from build123d import *

# Parameters (mm, degrees)
SKETCH_W        = 6
SKETCH_H        = 29
SKETCH_R        = 1.65
PAD_DEPTH       = 2.7
SKETCH001_W     = 4.5
SKETCH001_H     = 29
PAD001_DEPTH    = 1.5
SKETCH002_R     = 1.65
POCKET_DEPTH    = 5.701
CHAMFER_SIZE    = 0.4
CHAMFER001_SIZE = 0.4
FILLET_R        = 1
FILLET001_R     = 1


with BuildPart() as part:
    # Sketch → Pad (new body)
    with BuildSketch(Plane.XY):
        with Locations((-0.5, -9.5)):
            Rectangle(SKETCH_W, SKETCH_H)
        Circle(SKETCH_R, mode=Mode.SUBTRACT)
        with Locations((0, -10)):
            Circle(SKETCH_R, mode=Mode.SUBTRACT)
        with Locations((0, -20)):
            Circle(SKETCH_R, mode=Mode.SUBTRACT)
    extrude(amount=PAD_DEPTH)

    # Sketch001 (on Face8 of Pad) → Pad001 (join)
    with BuildSketch(Plane(origin=(0, 0, 0), x_dir=(1, 0, 0), z_dir=(0, 0, -1))):
        with Locations((-1.25, 9.5)):
            Rectangle(SKETCH001_W, SKETCH001_H)
    extrude(amount=PAD001_DEPTH)

    # Sketch002 → Pocket (cut, through all)
    with BuildSketch(Plane.XY.offset(4.2)):
        Circle(SKETCH002_R)
        with Locations((0, -10)):
            Circle(SKETCH002_R)
        with Locations((0, -20)):
            Circle(SKETCH002_R)
    extrude(amount=-POCKET_DEPTH, mode=Mode.SUBTRACT)

    # Chamfer
    chamfer_edges = [part.edges().sort_by_distance(p)[0] for p in [
        (2.5, -9.5, 0),
        (1, 3.15622, -1.5),
        (1, -5, -1.5),
        (1, -15, -1.5),
        (1, -22.65622, -1.5),
    ]]
    chamfer(chamfer_edges, length=CHAMFER_SIZE)

    # Chamfer001
    chamfer001_edges = [part.edges().sort_by_distance(p)[0] for p in [
        (-3.5, -9.5, -1.5),
    ]]
    chamfer(chamfer001_edges, length=CHAMFER001_SIZE)

    # Fillet
    fillet_edges = [part.edges().sort_by_distance(p)[0] for p in [
        (2.5, 5, 1.55),
        (1, 5, -0.55),
        (-3.5, 5, -0.55),
        (-3.5, 5, 1.35),
    ]]
    fillet(fillet_edges, radius=FILLET_R)

    # Fillet001
    fillet001_edges = [part.edges().sort_by_distance(p)[0] for p in [
        (2.5, -24, 1.55),
        (1, -24, -0.55),
        (-3.5, -24, -0.55),
        (-3.5, -24, 1.35),
    ]]
    fillet(fillet001_edges, radius=FILLET001_R)


solid = part.part
Can you work these out from the model? Positions are in its coordinate system, mm. A direction names the side the tool comes from. Coordinates: 2 decimals unless noted, no trailing zeros. Loops run counter-clockwise (first coordinate to the right, second up) from the corner with the lowest first, then second, coordinate; pieces in that order, holes last. Notation, with made-up numbers: (31.5, 38) - (65.5, 38) arc R19 cw to (65.5, 74) - close; hole circle Ø11 at (17.5, 20.25). An arc over 180 degrees is marked (long way). Put each result on its own line as item: value. Start each with the question number.
Item 1: Which directions (+Z, -Z, +X, -X, +Y, -Y) give clear straight access to the entire face, cutting with the end or side of a thin tool? Please do faces 5 (the face through (0.715, -23.699, -0.76)), 6 (the face through (1, 2.7, -0.5)), 7 (the face through (2.215, -23.699, 1.369)).
Item 2: Suppose I cut it at B-B (x = -0.6). Please give me the cut outline in (y, z), and give its area (3 significant figures).
Item 3: If we mould it in two halves opening along Y, with no side actions, what happens to faces 1 (the face through (0.699, 4.715, -0.76)), 2 (the face through (-3.215, -23.699, 0.629)), 3 (the face through (1, -4.9, -0.5)), 4 (the face through (-1.65, 0.07, 0.63))? For each: +Y half, -Y half, draft (parallel to the pull), parting line (faces both ways), or undercut.
Item 4: Suppose I cut it at D-D (y = -5). Please give me the cut outline in (x, z), and give its area (3 significant figures).
Item 5: Suppose I cut it at A-A (y = -10). Please give me the cut outline in (x, z), and give its area (4 significant figures).
Item 6: For pin 1 (0.6 mm diameter, centred on x = 1, y = -11.5, fed in from -Z); pin 2 (3 mm diameter, centred on x = 0, y = -10, fed in from -Z); pin 3 (1.2 mm diameter, centred on y = -22.5, z = -0.5, fed in from +X); pin 4 (1.2 mm diameter, centred on y = -5, z = -1, fed in from +X), each with a flat end and sliding along its axis, tell me the tip position at first contact or that it passes through.
Item 7: If I drill on line 1 along Y through (x, z) = (0, 1.4); line 2 along Y through (x, z) = (0.95, 1.6); line 3 along Z through (x, y) = (1.6, -6), over which ranges is the centre line in solid material (lowest first)?
Item 8: Suppose I cut it at C-C (z = -0.55). Please give me the cut outline in (x, y).
Here are the results:
1. face 5: -Z, +X, -Y
1. face 6: -Z, +X, +Y, -Y
1. face 7: +Z, -Z, +X, -Y
2. outline: (-24, -1.5) - (-21.54, -1.5) - (-21.54, 2.7) - (-24, 2.7) - close; (-18.46, -1.5) - (-11.54, -1.5) - (-11.54, 2.7) - (-18.46, 2.7) - close; (-8.46, -1.5) - (-1.54, -1.5) - (-1.54, 2.7) - (-8.46, 2.7) - close; (1.54, -1.5) - (5, -1.5) - (5, 2.7) - (1.54, 2.7) - close
2. area: 83.1 mm²
3. face 1: +Y half
3. face 2: -Y half
3. face 3: draft
3. face 4: undercut
4. outline: (-3.5, -1.1) - (-3.1, -1.5) - (0.6, -1.5) - (1, -1.1) - (1, 0) - (2.1, 0) - (2.5, 0.4) - (2.5, 2.7) - (-3.5, 2.7) - close
4. area: 22.7 mm²
5. outline: (-3.5, -1.1) - (-3.1, -1.5) - (-1.65, -1.5) - (-1.65, 2.7) - (-3.5, 2.7) - close; (1.65, 0) - (2.1, 0) - (2.5, 0.4) - (2.5, 2.7) - (1.65, 2.7) - close
5. area: 9.905 mm²
6. pin 1: z = -1.4
6. pin 2: through
6. pin 3: x = 2.2
6. pin 4: x = 1
7. line 1: -24 to -21.65, -18.35 to -11.65, -8.35 to -1.65, 1.65 to 5
7. line 2: -24 to -21.35, -18.65 to -11.35, -8.65 to -1.35, 1.35 to 5
7. line 3: 0 to 2.7
8. outline: (-3.5, -23) arc R1 ccw to (-2.5, -24) - (0, -24) arc R1 ccw to (1, -23) - (1, -21.31) arc R1.65 cw (long way) to (1, -18.69) - (1, -11.31) arc R1.65 cw (long way) to (1, -8.69) - (1, -1.31) arc R1.65 cw (long way) to (1, 1.31) - (1, 4) arc R1 ccw to (0, 5) - (-2.5, 5) arc R1 ccw to (-3.5, 4) - close
